from build123d import *

# Parameters (mm, degrees)
SKETCH7_W               = 4.7625
SKETCH7_H               = 2.12122512
BOSS_EXTRUDE2_DEPTH     = 130.175
SKETCH8_W               = 2.12122512
SKETCH8_H               = 4.7625
BOSS_EXTRUDE3_DEPTH     = 130.175
BOSS_EXTRUDE4_DEPTH     = 130.175
CUT_EXTRUDE1_DEPTH      = 150.236313895
CUT_EXTRUDE1_DEPTH_BACK = 12.241080233


with BuildPart() as part:
    # Sketch7 → Boss-Extrude2 (new body, symmetric)
    with BuildSketch(Plane.XY):
        with Locations((-4.92125, -2.560612608)):
            Rectangle(SKETCH7_W, SKETCH7_H)
    extrude(amount=BOSS_EXTRUDE2_DEPTH, both=True)

    # Sketch8 → Boss-Extrude3 (add, symmetric)
    with BuildSketch(Plane.XY):
        with Locations((-2.560612608, -4.92125)):
            Rectangle(SKETCH8_W, SKETCH8_H)
    extrude(amount=BOSS_EXTRUDE3_DEPTH, both=True)

    # Sketch11 → Boss-Extrude4 (add, symmetric)
    with BuildSketch(Plane.XY):
        with BuildLine():
            Line((-2.54, 1.500000048), (-2.54, -1.500000048))
            Line((-2.54, -1.500000048), (-7.3025, -1.500000048))
            Line((-7.3025, -1.500000048), (-7.3025, -3.621225168))
            Line((-7.3025, -3.621225168), (-5.866289198, -3.621225168))
            Line((-5.866289198, -3.621225168), (-3.621225168, -5.866289198))
            Line((-3.621225168, -5.866289198), (-3.621225168, -7.3025))
            Line((-3.621225168, -7.3025), (-1.500000048, -7.3025))
            Line((-1.500000048, -7.3025), (-1.500000048, -2.54))
            Line((-1.500000048, -2.54), (1.500000048, -2.54))
            Line((1.500000048, -2.54), (1.500000048, -0.519999976))
            ThreePointArc((1.500000048, -0.519999976), (0.908355739, 0.908355739), (-0.519999976, 1.500000048))
            Line((-0.519999976, 1.500000048), (-2.54, 1.500000048))
        make_face()
    extrude(amount=BOSS_EXTRUDE4_DEPTH, both=True)

    # Sketch17 → Cut-Extrude1 (cut, two sides)
    with BuildSketch(Plane(origin=(0, 0, 113.704878), x_dir=(0.707106781, 0, -0.707106781), z_dir=(-0.577350269, -0.577350269, -0.577350269))) as cut_extrude1_sk:
        Polygon((9.347296833, 5.396664343), (0, 0), (0, -10.793328686), (-219.970452561, 116.206671314), (-210.623155728, 132.396664343), align=None)
    extrude(amount=CUT_EXTRUDE1_DEPTH, mode=Mode.SUBTRACT)
    extrude(cut_extrude1_sk.sketch, amount=-CUT_EXTRUDE1_DEPTH_BACK, mode=Mode.SUBTRACT)


solid = part.part
Source: CAD feature listing. Evaluate the final solid. Frame: model axes, mm. A direction names the side the tool comes from. Coordinates: 2 decimals unless noted, no trailing zeros. Order: outer loops, then holes, each group sorted by start corner. A loop starts at its lowest first (then second) coordinate and runs counter-clockwise, first axis right, second up. Notation, with made-up numbers: M 2,-1.5 L 17,-1.5 A31 cw 17,28.5 Z; hole C 59,2.25 d2. An arc over 180 degrees is marked long. Write each question's results on one line, items separated by ' | '. Start each with the question number.
Item 1: Line query: probe 1 along Y at (x, z) = (-7, 72.5); probe 2 along X at (y, z) = (-0.75, 90). Output: solid intervals per line, ascending.
Item 2: First-contact query: pin 1 Ø0.9 at (y, z) = (0, 21.5) entering from -X; pin 2 Ø3 at (x, y) = (-1, -5.5) entering from +Z; pin 3 Ø2.5 at (y, z) = (-5, -50.5) entering from +X. Flat tips, straight axial feed; report the tip coordinate or a pass-through.
Item 3: Cut plane A-A (z = -107.5). Return loops of the section in (x, y), and give its area (3 significant figures).
Item 4: Set-up query: faces 1 (the face through (-3, -3, -130.175)), 2 (the face through (-1.5, -5, -8)), 3 (the face through (-5, -1.5, -8)). Return all of +Z, -Z, +X, -X, +Y, -Y with unobstructed straight access to the full face (end or side cutting, diameter ignored); none if empty.
Checked values:
1) probe 1: y = -3.62 to -1.5 | probe 2: x = -2.54 to 1.5
2) pin 1: stops at x = -2.54 | pin 2: stops at z = 109.62 | pin 3: stops at x = -1.5
3) outline: M -7.3,-3.62 L -5.87,-3.62 L -3.62,-5.87 L -3.62,-7.3 L -1.5,-7.3 L -1.5,-2.54 L 1.5,-2.54 L 1.5,-0.52 A2.02 ccw -0.52,1.5 L -2.54,1.5 L -2.54,-1.5 L -7.3,-1.5 Z | area: 37.0 mm2
4) face 1: -Z, +X, -X, +Y, -Y | face 2: +Z, -Z, +X, -Y | face 3: +Z, -Z, -X, +Y
